For this review, take the finished solid that the model builds, in its own axes (mm). Face numbers are marked on the shaded views. A direction names the side the tool comes from. Give positions to 0.01 mm unless a question says otherwise; leave off trailing zeros. Loops run counter-clockwise (first coordinate to the right, second up) from the corner with the lowest first, then second, coordinate; pieces in that order, holes last.
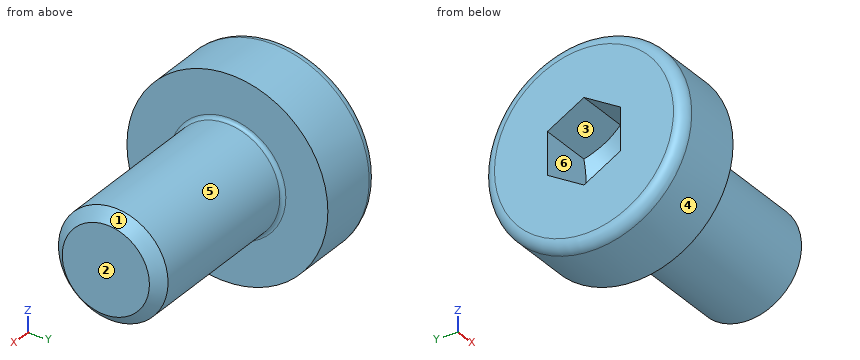
Autodesk Inventor part; units mm, degrees
ref_plane "Work Plane1" through (29, 0, 0) normal (0, -1, 0) x (1, 0, 0)
ref_plane "YZ Plane" through (0, 0, 0) normal (1, 0, 0) x (0, 1, 0)
ref_plane "XZ Plane" through (0, 0, 0) normal (0, 1, 0) x (-1, 0, 0)
sketch "Sketch1" plane through (0, 0, 0) normal (0, 0, 1) x (1, 0, 0)
  line L0 (0.1667, 0) -> (5, 0)
  line L1 (5, 0) -> (5, 1.5)
  line L2 (5, 1.5) -> (1.5, 1.5)
  line L3 (1.5, 1.5) -> (1.1932, 1.5)
  line L4 (1.1932, 1.5) -> (0, 1.5)
  line L5 (0, 1.5) -> (0, 2.75)
  line L6 (0, 2.75) -> (-2, 2.75)
  line L7 (-2, 2.75) -> (-2, 1.1547)
  line L8 (-2, 1.1547) -> (-0.5, 1.1547)
  line L9 (-0.5, 1.1547) -> (0.1667, 0)
  line L10 (-3.4, 0) -> (6.4, 0)
  line L11 (0, -0.55) -> (0, 3.3)
  line L12 (1.5, 1.5) -> (0, 1.5) construction
  dimension "d1" = 3.5
  dimension "d2" = 0.3068
  dimension "d3" = 2
  dimension "d4" = 1.5
  dimension "d5" = 60
  dimension "d6" = 3
  dimension "d7" = 3
  dimension "d8" = 2.3094
  dimension "d9" = 5.5
  dimension "d26" = 5
revolve "Body" add sketch "Sketch1" angle 360 about axis through (0.1667, 0, 0) along (1, 0, 0) contours L9 L11 L4 L3 L2 L1 L0 | L9 L8 L7 L6 L5 L11
sketch "Sketch2" plane through (-2, 0, 0) normal (-1, 0, 0) x (0, 0, 1)
  circle A0 centre (0, 0) radius 1.1547
  line L0 (0, -3.85) -> (0, 3.85)
  line L1 (-3.85, 0) -> (3.85, 0)
  line L2 (1.1547, 0) -> (0.5774, -1)
  line L3 (0.5774, -1) -> (-0.5774, -1)
  line L4 (-0.5774, -1) -> (-1.1547, 0)
  line L5 (-1.1547, 0) -> (-0.5774, 1)
  line L6 (-0.5774, 1) -> (0.5774, 1)
  line L7 (0.5774, 1) -> (1.1547, 0)
extrude "Slot" add sketch "Sketch2" against normal up to next contours L7 A0 | A0 L2 | L6 L0 A0 | A0 L0 L3 | L0 L6 A0 | A0 L3 L0 | L4 A0 | A0 L5
fillet "Fillet1" radius 0.3 1 edges at (-2, -2.75, 0)
thread "Thread"
chamfer "Chamfer1" distance 0.3067 distance2 0.3067 1 edges at (5, -1.5, 0) measured on face at (5, -0.2617, -0.7882)
ref_plane "Work Plane1" through (29, 0, 0) normal (0, -1, 0) x (1, 0, 0)
fillet "Fillet2" radius 0.1 1 edges at (0, -1.5, 0)
equation "\"d1\" = GEL"
equation "\"d3\" = KOH"
equation "\"d4\" = INTI"
equation "\"d6\" = GD"
equation "\"d7\" = BDM"
equation "\"d8\" = 1.1547 * SW"
equation "\"d9\" = KOD"
equation "\"d26\" = NLG"
equation "\"d30\" = R"
equation "\"d17\" = RR"
equation "\"d13\" = GEL"
equation "\"d15\" = -0.5 * SPD + 0.5 * GD"
equation "\"d16\" = GUL"
equation "\"GD\" = NND"
equation "\"NLG\" = 5"
equation "\"GEL\" = 3.5"
equation "\"KOD\" = 5.5"
equation "\"KOH\" = 2"
equation "\"INTI\" = 1.5"
equation "\"GAL\" = 0.61345 * PTC"
equation "\"GUL\" = 0.61345 * PTC"
equation "\"BDM\" = NND"
equation "\"SW\" = 2"
equation "\"RR\" = 0.3"
equation "\"SPD\" = NND - 1.2269 * PTC"
equation "\"R\" = 0.1"
equation "\"TOA\" = 30deg"
equation "\"GD1\" = THREADDIA - 1.2269 * PTC"
equation "\"THREADDIA\" = 3"
equation "\"FAWI\" = 45deg"
equation "\"ANG\" = 120deg"
equation "\"PTC\" = 0.5"
equation "\"NND\" = 3"
equation "\"E0\" = 1.155 * SW"
properties part number "DIN 7984 - M3 x 5" material "Steel, Mild"
Item 1: For L1, parallel to X at y = 2.15, z = -1.05; L2, parallel to Z at x = -0.25, y = 0.4; L3, parallel to Z at x = 0.5, y = 0.7, list the stretches that pass through material, from the lowest coordinate up.
Answer:
L1: x = -2 to 0
L2: z = -2.72 to -0.6, 0.6 to 2.72
L3: z = -1.33 to 1.33
Item 2: Tool access review of the marked faces 4, 5 and 6: name each direction out of +Z, -Z, +X, -X, +Y, -Y from which nothing blocks a thin tool from reaching the whole face with its end or side.
Answer:
face 4: +X, -X
face 5: +X
face 6: -X
Item 3: The part is to be moulded in two halves that separate along Y. For the marked faces 1, 2 and 3, say which applies: released by +Y, released by -Y, zero draft, split by the parting line, or undercut.
Answer:
face 1: split by the parting line
face 2: zero draft
face 3: undercut
Item 4: Take a section at A-A on x = 0.75. Give the boundary of the cut face in (y, z).
Answer:
outline: circle Ø3 at (0, 0)
